Drawing for the job (mm, zero at the part's lowest x, y, z). Coordinates: 2 decimals unless noted, no trailing zeros. Order: outer loops, then holes, each group sorted by start corner. A loop starts at its lowest first (then second) coordinate and runs counter-clockwise, first axis right, second up. Notation, with made-up numbers: (42.5, 85.25) -> (93.5, 85.25) arc R14 ccw to (93.5, 90.25) -> close; hole circle Ø10 at (-10, 19.25). An arc over 180 degrees is marked (long way). Write each question's results on one line, items separated by ' | '.
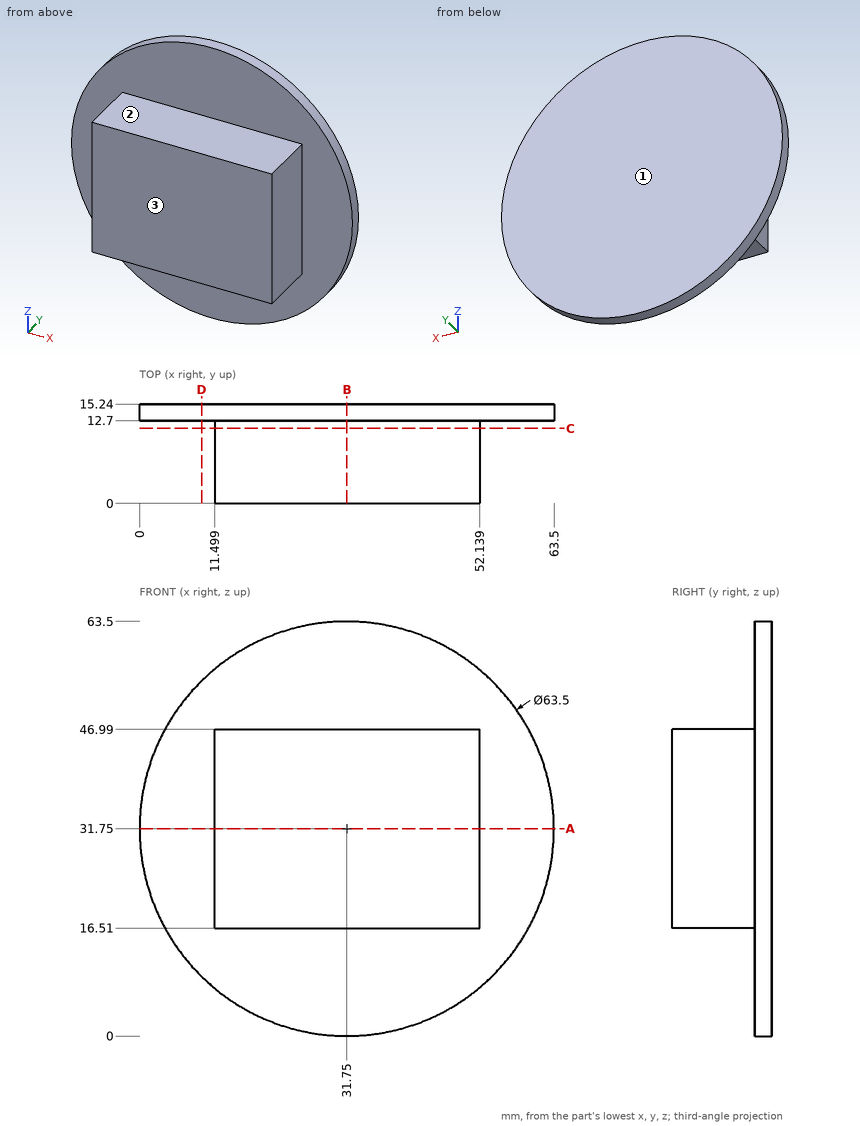
Item 1: Pull direction Y, two halves, no side cores. Call the marked faces 1, 2 and 3: released by +Y, released by -Y, zero draft, split by the parting line, or undercut.
Answer:
face 1: released by +Y | face 2: zero draft | face 3: released by -Y
Item 2: Drill centre lines: line 1 (Z direction, x = 15.5, y = 4); line 2 (Y direction, x = 40.5, z = 9); line 3 (X direction, y = 12.5, z = 36). Where is each one in solid material? Low to high. Write a range as from..to.
Answer:
line 1: z = 16.51..46.99 | line 2: y = 12.7..15.24 | line 3: x = 11.5..52.14
Item 3: Slice it at C-C, the plane y = 11.5. List the corners of the cut face in (x, z).
Answer:
outline: (11.5, 16.51) -> (52.14, 16.51) -> (52.14, 46.99) -> (11.5, 46.99) -> close
Item 4: Slice it at A-A, the plane z = 31.75. List the corners of the cut face in (x, y), and give its area (3 significant figures).
Answer:
outline: (0, 12.7) -> (11.5, 12.7) -> (11.5, 0) -> (52.14, 0) -> (52.14, 12.7) -> (63.5, 12.7) -> (63.5, 15.24) -> (0, 15.24) -> close | area: 677 mm^2
Item 5: Slice it at B-B, the plane x = 31.75. List the corners of the cut face in (y, z), and give its area (3 significant figures).
Answer:
outline: (0, 16.51) -> (12.7, 16.51) -> (12.7, 0) -> (15.24, 0) -> (15.24, 63.5) -> (12.7, 63.5) -> (12.7, 46.99) -> (0, 46.99) -> close | area: 548 mm^2
Item 6: Pin check, flat tips, straight feed: pin 1 (6.5 mm diameter, centred on x = 27.5, y = 5.5, fed in from -Z); pin 2 (3 mm diameter, centred on x = 42, y = 10.5, fed in from +Z); pin 3 (3 mm diameter, centred on y = 6, z = 32.5, fed in from +X). Stop position of each tip, or through.
Answer:
pin 1: stops at z = 16.51 | pin 2: stops at z = 46.99 | pin 3: stops at x = 52.14
Item 7: Slice it at D-D, the plane x = 9.5. List the corners of the cut face in (y, z), and give its area (3 significant figures).
Answer:
outline: (12.7, 9.1) -> (15.24, 9.1) -> (15.24, 54.4) -> (12.7, 54.4) -> close | area: 115 mm^2
